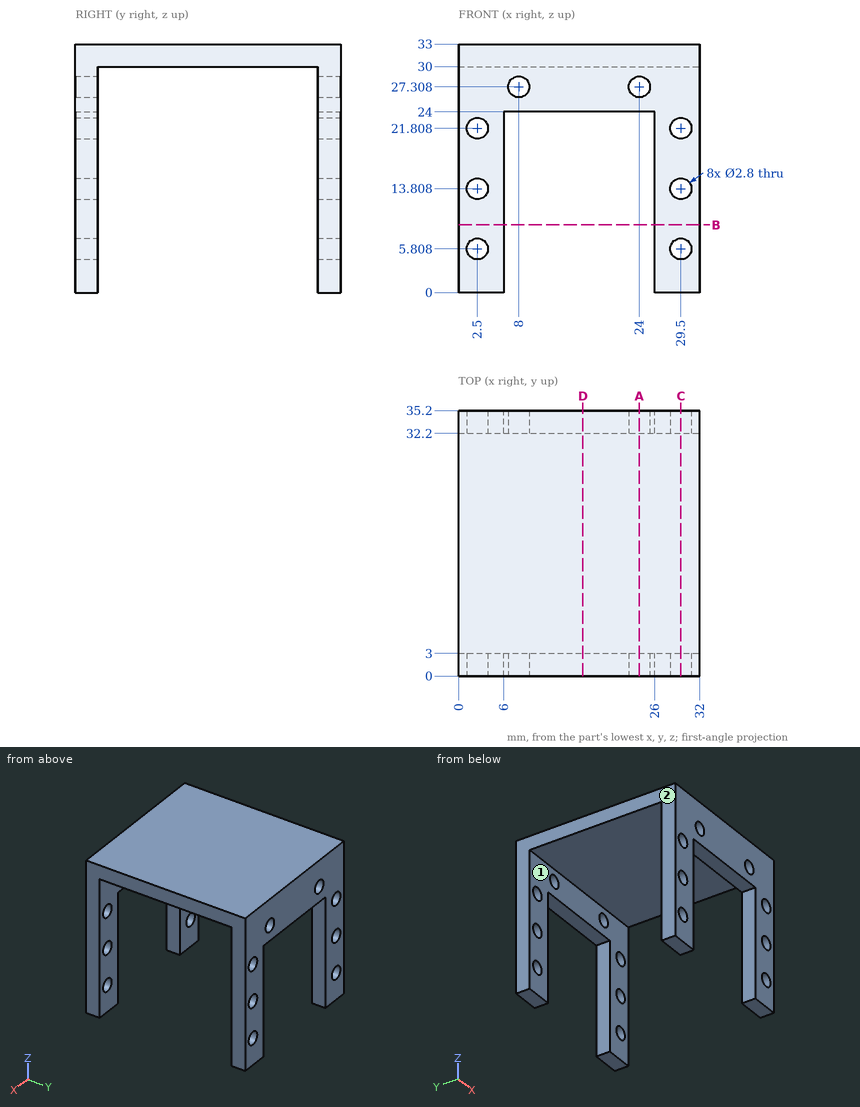
Here's the drawing with two shaded views (mm, measured from the low corner). I have some questions. A direction names the side the tool comes from. Coordinates: 2 decimals unless noted, no trailing zeros. Write each loop counter-clockwise with the first axis right and the second up, starting at its lowest first coordinate (ties: lowest second). Pieces come first, ordered by that corner, then holes. Notation, with made-up numbers: (85.25, -8.75) -> (132.25, -8.75) arc R26 ccw to (132.25, 24.25) -> close; hole circle Ø10 at (-14, 67.5). An arc over 180 degrees is marked (long way). Write item = value, one per line. Start each with the question number.
(1) I want a section at C-C (x = 29.5). Give the number of separate pieces and of enclosed holes in the cut face, plus the area to 3 significant figures.
(2) I want a section at B-B (z = 9). Please give me the cut outline in (x, y).
(3) I need wall thicknesses on line 1 (Z direction, x = 29.5, y = 33.05); line 2 (Y direction, x = 4.5, z = 25.5); line 3 (Z direction, x = 24, y = 2.2). Which ranges of each line are inside material? Lowest first, please. Write a range as [from, to].
(4) I want a section at D-D (x = 16.5). Please give me the cut outline in (y, z).
(5) Which directions (+Z, -Z, +X, -X, +Y, -Y) give clear straight access to the entire face, cutting with the end or side of a thin tool? Please do the marked faces 1 and 2.
(6) I want a section at A-A (x = 24). Please give me the cut outline in (y, z).
(7) Will these pins go through, and if not, where does the flat tip stop? pin 1 (1.7 mm diameter, centred on x = 2.5, z = 5.81, fed in from -Y); pin 2 (1.5 mm diameter, centred on x = 15.5, y = 34.5, fed in from -Z); pin 3 (8 mm diameter, centred on x = 9, y = 14.5, fed in from -Z).
Result set:
q1.separate_pieces = 7
q1.enclosed_holes = 0
q1.area = 235 mm2
q2.outline = (0, 0) -> (6, 0) -> (6, 3) -> (0, 3) -> close; (0, 32.2) -> (6, 32.2) -> (6, 35.2) -> (0, 35.2) -> close; (26, 0) -> (32, 0) -> (32, 3) -> (26, 3) -> close; (26, 32.2) -> (32, 32.2) -> (32, 35.2) -> (26, 35.2) -> close
q3.line_1 = [0, 4.41], [7.21, 12.41], [15.21, 20.41], [23.21, 33]
q3.line_2 = [0, 3], [32.2, 35.2]
q3.line_3 = [24, 25.91], [28.71, 33]
q4.outline = (0, 24) -> (3, 24) -> (3, 30) -> (32.2, 30) -> (32.2, 24) -> (35.2, 24) -> (35.2, 33) -> (0, 33) -> close
q5.face_1 = -Z, +X, -X
q5.face_2 = +Z, -Z, -X, +Y, -Y
q6.outline = (0, 24) -> (3, 24) -> (3, 25.91) -> (0, 25.91) -> close; (0, 28.71) -> (3, 28.71) -> (3, 30) -> (32.2, 30) -> (32.2, 28.71) -> (35.2, 28.71) -> (35.2, 33) -> (0, 33) -> close; (32.2, 24) -> (35.2, 24) -> (35.2, 25.91) -> (32.2, 25.91) -> close
q7.pin_1 = through
q7.pin_2 = 24
q7.pin_3 = 30
